from build123d import *

# Parameters (mm, degrees)
SKETCH1_W           = 127
SKETCH1_H           = 10
BOSS_EXTRUDE1_DEPTH = 10
BOSS_EXTRUDE2_DEPTH = 10
FILLET1_R           = 2
CUT_EXTRUDE1_REACH  = 12


with BuildPart() as part:
    # Sketch1 → Boss-Extrude1 (new body)
    with BuildSketch(Plane(origin=(0, 0, 0), x_dir=(1, 0, 0), z_dir=(0, 1, 0))):
        Rectangle(SKETCH1_W, SKETCH1_H)
    extrude(amount=BOSS_EXTRUDE1_DEPTH)

    # Sketch2 → Boss-Extrude2 (add)
    with BuildSketch(Plane(origin=(0, 10, 0), x_dir=(1, 0, 0), z_dir=(0, 1, 0))):
        Polygon((-63.5, 5), (-63.5, 17), (-51.5, 5), align=None)
        Polygon((51.5, 5), (63.5, 5), (63.5, 17), align=None)
    extrude(amount=-BOSS_EXTRUDE2_DEPTH)

    # Fillet1
    fillet1_edges = [part.edges().sort_by_distance(p)[0] for p in [
        (-51.5, 5, -5),
        (-63.5, 5, -17),
        (51.5, 5, -5),
        (63.5, 5, -17),
        (63.5, 5, 5),
        (-63.5, 5, 5),
    ]]
    fillet(fillet1_edges, radius=FILLET1_R)

    # Sketch4 → Cut-Extrude1 (cut, up to next)
    with BuildSketch(Plane(origin=(0, 10, 0), x_dir=(1, 0, 0), z_dir=(0, 1, 0)), mode=Mode.PRIVATE) as cut_extrude1_sk1:
        with BuildLine():
            Line((-50, 2), (50, 2))
            ThreePointArc((50, 2), (52, 0), (50, -2))
            Line((50, -2), (-50, -2))
            ThreePointArc((-50, -2), (-52, 0), (-50, 2))
        make_face()
    cut_extrude1_tool1 = extrude(cut_extrude1_sk1.sketch, amount=-CUT_EXTRUDE1_REACH, mode=Mode.PRIVATE) & part.part
    add(cut_extrude1_tool1.solids().sort_by_distance((0, 10, 0))[0], mode=Mode.SUBTRACT)


solid = part.part
CAD build for the part. Positions are in the model's coordinates, mm. A direction names the side the tool comes from. Round coordinates to 2 decimals unless told otherwise and drop trailing zeros. Write each loop counter-clockwise with the first axis right and the second up, starting at its lowest first coordinate (ties: lowest second). Pieces come first, ordered by that corner, then holes.
(1) Slice it at A-A, the plane z = -7. Write the cut outline in (x, y).
(2) Slice it at D-D, the plane x = 55.5. Write the cut outline in (y, z).
(3) Slice it at C-C, the plane y = 5.25. Write the cut outline in (x, z).
(4) Probe line 1 along Z through (x, y) = (-35, 2.5); line 2 along X through (y, z) = (8.5, -5.5); line 3 along X through (y, z) = (1.75, 1.5). List the from-to ranges inside material, lowest first.
(5) 3-axis set-ups, long thin cutter, end or side, ignore diameter. For faces 5 (the face through (1, 0, -3)), 6 (the face through (56.1, 5.1, -9.6)), 7 (the face through (52, 5, 0)): which of +Z, -Z, +X, -X, +Y, -Y reach the whole face in a straight line?
(6) Mould opens along Z. For faces 1 (the face through (63.5, 5, -4)), 2 (the face through (-1, 5, -2)), 3 (the face through (-52, 5, 0)), 4 (the face through (62.93, 5.07, 4.4)) say: pulls with the +Z half, pulls with the -Z half, needs draft (parallel to the pull), parting line crosses it, or undercut.
(7) Slice it at B-B, the plane x = 37. Write the cut outline in (y, z).
(8) Drop a flat-ended pin along its axis: P1, Ø6, axis at x = 39.5, y = 6.5, coming from the -Z side. Give the stop position or say it passes through.
From the geometry:
1. outline: (-63.5, 0) - (-53.5, 0) - (-53.5, 10) - (-63.5, 10) - close; (53.5, 0) - (63.5, 0) - (63.5, 10) - (53.5, 10) - close
2. outline: (0, -9) - (10, -9) - (10, 5) - (0, 5) - close
3. outline: (-63.5, -12.17) arc R2 ccw to (-60.09, -13.59) - (-52.09, -5.59) arc R2 cw to (-50.67, -5) - (50.67, -5) arc R2 cw to (52.09, -5.59) - (60.09, -13.59) arc R2 ccw to (63.5, -12.17) - (63.5, 3) arc R2 ccw to (61.5, 5) - (-61.5, 5) arc R2 ccw to (-63.5, 3) - close; hole (-50, -2) - (50, -2) arc R2 ccw to (50, 2) - (-50, 2) arc R2 ccw to start
4. line 1: z = -5 to -2, 2 to 5
4. line 2: x = -63.5 to -51.99, 51.99 to 63.5
4. line 3: x = -63.5 to -51.32, 51.32 to 63.5
5. face 5: +Z, -Z, +X, -X, -Y
5. face 6: -Z, +Y, -Y
5. face 7: +Y, -Y
6. face 1: needs draft
6. face 2: undercut
6. face 3: undercut
6. face 4: pulls with the +Z half
7. outline: (0, -5) - (10, -5) - (10, -2) - (0, -2) - close; (0, 2) - (10, 2) - (10, 5) - (0, 5) - close
8. P1: stops at z = -5
